Could you check a few things on this model? Use its own coordinates, in mm. A direction names the side the tool comes from. Round coordinates to 2 decimals unless told otherwise and drop trailing zeros. Loops run counter-clockwise (first coordinate to the right, second up) from the corner with the lowest first, then second, coordinate; pieces in that order, holes last. Notation, with made-up numbers: (16.25, -34) -> (73.25, -34) arc R16 cw to (73.25, -25) -> close; hole circle Ø11 at (66.25, -32). An arc over 180 degrees is marked (long way). Write each question's results on one line, items separated by ' | '. Start each with the question number.
1) If I drill on probe 1 along Y at (x, z) = (35, -21.5); probe 2 along X at (y, z) = (8.4, -40); probe 3 along X at (y, z) = (4.25, 40), over which ranges is the centre line in solid material (lowest first)?
2) Imagine slicing it at A-A, the plane z = 0. List the corners of the cut face in (x, y) for me, plus the area to 3 significant figures.
3) Which directions (+Z, -Z, +X, -X, +Y, -Y) give clear straight access to the entire face, cutting with the end or side of a thin tool? Please do faces 4 (the flat face through (-10, 35, 5)), 5 (the flat face through (-0.517, 4.93, 35.938)), 6 (the cylindrical face through (34.41, 8.99, -38.37)).
4) Imagine slicing it at C-C, the plane x = -40.5. List the corners of the cut face in (y, z) for me.
5) For P1, Ø2.5, axis at x = -46, y = 34, coming from the +Z side; P2, Ø8.5, axis at x = -11, y = 36, coming from the -Z side; P3, Ø4, axis at x = -47, z = 0.5, coming from the +Y side, each with a flat end and sliding along its axis, tell me the tip position at first contact or that it passes through.
6) We'd pull the mould along X, two halves only. Please class faces 1 (the cylindrical face through (48.81, 4.93, 50.3)), 2 (the flat face through (-29, 40, 16)), 3 (the cylindrical face through (49.05, 8.99, 38.37)): pulls with the +X half, pulls with the -X half, needs draft (parallel to the pull), parting line crosses it, or undercut.
7) Imagine slicing it at D-D, the plane y = 22.5. List the corners of the cut face in (x, z) for me.
8) Imagine slicing it at B-B, the plane y = 31.5. List the corners of the cut face in (x, z) for me, plus the area to 3 significant figures.
Autodesk Inventor part; units mm, degrees
ref_plane "YZ Plane" through (0, 0, 0) normal (1, 0, 0) x (0, 1, 0)
ref_plane "XZ Plane" through (0, 0, 0) normal (0, 1, 0) x (-1, 0, 0)
ref_plane "XY Plane" through (0, 0, 0) normal (0, 0, 1) x (1, 0, 0)
sketch "Sketch1" plane through (0, 0, 0) normal (0, 1, 0) x (-1, 0, 0)
  arc A0 (36.9231, -20.7692) -> (36.9231, 20.7692) centre (28.2692, 0) ccw
  line L0 (36.9231, 20.7692) -> (-36.9231, 51.5385)
  line L1 (36.9231, -20.7692) -> (-36.9231, -51.5385)
  arc A1 (-36.9231, 51.5385) -> (-54.2308, 40) centre (-41.7308, 40) ccw
  arc A2 (-54.2308, -40) -> (-36.9231, -51.5385) centre (-41.7308, -40) ccw
  line L2 (72.3868, 0) -> (-78.9359, 0)
  line L3 (0, -78.6378) -> (0, 78.6378)
  line L4 (-54.2308, 40) -> (-54.2308, -40)
  point P0 (0, 0)
  point P1 (0, -36.1538)
  point P2 (0, 36.1538)
  point P3 (-54.2308, 0)
  dimension "d0" = 70
  dimension "d1" = 80
  dimension "d2" = 12.5
  dimension "d3" = 45
extrude "Extrusion1" add sketch "Sketch1" along normal blind 10
sketch "Sketch2" plane through (0, 10, 0) normal (0, 1, 0) x (1, 0, 0)
  line L0 (-36.9231, -20.7692) -> (36.9231, -51.5385)
  arc A0 (36.9231, -51.5385) -> (54.2308, -40) centre (41.7308, -40) ccw
  line L1 (54.2308, -40) -> (54.2308, 40)
  arc A1 (54.2308, 40) -> (36.9231, 51.5385) centre (41.7308, 40) ccw
  line L2 (36.9231, 51.5385) -> (-36.9231, 20.7692)
  arc A2 (-36.9231, 20.7692) -> (-36.9231, -20.7692) centre (-28.2692, 0) ccw
  circle A3 centre (-28.2692, 0) radius 22.5
  point P0 (0, 0)
extrude "Extrusion2" add sketch "Sketch2" along normal blind 30 contours A2 A3
sketch "Sketch3" plane through (-28.2692, 40, 0) normal (0, 1, 0) x (1, 0, 0)
  circle A0 centre (0, 0) radius 15
  point P0 (28.2692, 0)
  dimension "d8" = 30
extrude "Extrusion3" cut sketch "Sketch3" against normal through all
sketch "Sketch4" plane through (-28.2692, 40, 0) normal (0, 1, 0) x (1, 0, 0)
  line L0 (-24.7308, -5) -> (25.2692, -5)
  line L1 (25.2692, -5) -> (25.2692, 5)
  line L2 (25.2692, 5) -> (-24.7308, 5)
  line L3 (-24.7308, 5) -> (-24.7308, -5)
  line L4 (-59.7, 0) -> (106.2, 0)
  line L5 (28.2692, 73.5) -> (28.2692, -73.5)
  point P0 (28.2692, 0)
  point P1 (-24.7308, 0)
  dimension "d14" = 10
  dimension "d15" = 50
  dimension "d16" = 3
extrude "Extrusion4" cut sketch "Sketch4" against normal blind 10
hole "Hole1" at (41.7308, 10, 40) direction (0, -1, 0) diameter 10 end through all counterbore diameter 15 counterbore depth 2
mirror "Mirror1" about plane through (0, 0, 0) normal (0, 0, 1) of "Hole1"
properties part number "Workshop_1_Soln" material "Bronze, Soft Tin"
Checked values:
1) probe 1: 0 to 10 | probe 2: 9.23 to 34.23, 49.23 to 54.23 | probe 3: 9.23 to 36.73, 46.73 to 54.23
2) outline: (-50.77, 0) -> (-43.27, 0) -> (-43.27, 30) -> (-50.77, 30) -> close; (-13.27, 0) -> (54.23, 0) -> (54.23, 10) -> (-5.77, 10) -> (-5.77, 30) -> (-13.27, 30) -> close | area: 1,050 mm^2
3) face 4: +X, -X, +Y | face 5: +Z, -X, +Y, -Y | face 6: +Y
4) outline: (0, -18.89) -> (40, -18.89) -> (40, -8.68) -> (0, -8.68) -> close; (0, 8.68) -> (40, 8.68) -> (40, 18.89) -> (0, 18.89) -> close
5) P1: z = 15.32 | P2: z = -18.35 | P3: y = 30
6) face 1: parting line crosses it | face 2: needs draft | face 3: undercut
7) outline: circle Ø45 at (-28.27, 0); hole circle Ø30 at (-28.27, 0)
8) outline: (-50.21, -5) arc R22.5 ccw to (-36.92, -20.77) arc R22.5 ccw to (-6.33, -5) -> (-14.13, -5) arc R15 cw to (-42.41, -5) -> close; (-50.21, 5) -> (-42.41, 5) arc R15 cw to (-14.13, 5) -> (-6.33, 5) arc R22.5 ccw to start | area: 732 mm^2
